from build123d import *

# Parameters (mm, degrees)
BOSS_EXTRU_1_DEPTH      = 12
BOSS_EXTRU_1_DEPTH_BACK = 12
ENL_V_START             = 9
ESQUISSE2_R             = 1
ENL_V_MAT_EXTRU_1_DEPTH = 4
CONG_1_R                = 1
ESQUISSE3_R             = 1
ENL_V_MAT_EXTRU_2_DEPTH = 2.5
ENL_V_START_2           = -2.5
ESQUISSE6_R             = 1
ENL_V_MAT_EXTRU_4_DEPTH = 2.5


with BuildPart() as part:
    # Esquisse1 → Boss.-Extru.1 (new, two sides: drawn at the far end of the back side and taken through both)
    with BuildSketch(Plane.XY.offset(-BOSS_EXTRU_1_DEPTH_BACK)):
        with BuildLine():
            Line((11, -9), (2.692582404, -9))
            ThreePointArc((2.692582404, -9), (0, 5.5), (-2.692582404, -9))
            Line((-2.692582404, -9), (-11, -9))
            Line((-11, -9), (-11, 9))
            Line((-11, 9), (11, 9))
            Line((11, 9), (11, -9))
        make_face()
    extrude(amount=BOSS_EXTRU_1_DEPTH + BOSS_EXTRU_1_DEPTH_BACK)

    # Esquisse2 → Enlèv. mat.-Extru.1 (cut)
    with BuildSketch(Plane(origin=(0, 0, 0), x_dir=(1, 0, 0), z_dir=(0, 1, 0)).offset(ENL_V_START)):
        with Locations(Location((-7, 8, 0), (0, 0, 270))):
            Circle(ESQUISSE2_R)
        with Locations(Location((7, 8, 0), (0, 0, 270))):
            Circle(ESQUISSE2_R)
        with Locations(Location((7, -8, 0), (0, 0, 270))):
            Circle(ESQUISSE2_R)
        with Locations(Location((-7, -8, 0), (0, 0, 270))):
            Circle(ESQUISSE2_R)
    extrude(amount=-ENL_V_MAT_EXTRU_1_DEPTH, mode=Mode.SUBTRACT)

    # Congé1
    cong_1_edges = [part.edges().sort_by_distance(p)[0] for p in [
        (-11, 9, 0),
        (11, 9, 0),
        (11, -9, 0),
        (2.692582404, -9, 0),
        (-2.692582404, -9, 0),
        (-11, -9, 0),
        (0, 5.5, -12),
        (6.846291202, -9, -12),
        (-11, 0, 12),
        (-6.846291202, -9, 12),
        (0, 5.5, 12),
        (6.846291202, -9, 12),
        (11, 0, 12),
        (0, 9, 12),
        (11, 0, -12),
        (0, 9, -12),
        (-11, 0, -12),
        (-6.846291202, -9, -12),
    ]]
    fillet(cong_1_edges, radius=CONG_1_R)

    # Esquisse3 → Enlèv. mat.-Extru.2 (cut)
    with BuildSketch(Plane.ZY.offset(11)):
        with Locations((0, 5.5)):
            Circle(ESQUISSE3_R)
        with Locations((0, -5.5)):
            Circle(ESQUISSE3_R)
    extrude(amount=-ENL_V_MAT_EXTRU_2_DEPTH, mode=Mode.SUBTRACT)

    # Esquisse6 → Enlèv. mat.-Extru.4 (cut)
    with BuildSketch(Plane(origin=(11, 0, 0), x_dir=(0, 0, -1), z_dir=(1, 0, 0)).offset(ENL_V_START_2)):
        with Locations(Location((0, 5.5, 0), (0, 0, 180))):
            Circle(ESQUISSE6_R)
        with Locations(Location((0, -5.5, 0), (0, 0, 180))):
            Circle(ESQUISSE6_R)
    extrude(amount=ENL_V_MAT_EXTRU_4_DEPTH, mode=Mode.SUBTRACT)


solid = part.part
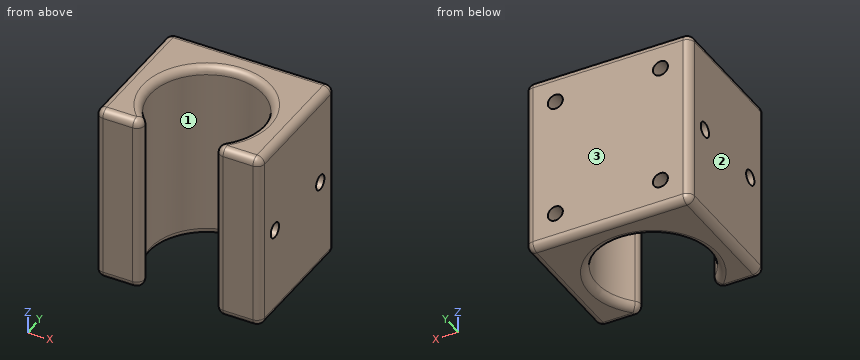
Check sheet for the modelled part. Datum: model origin and axes. Units: mm. Face numbers are marked on the shaded views. Coordinates: 2 decimals unless noted, no trailing zeros. Loops run counter-clockwise (first coordinate to the right, second up) from the corner with the lowest first, then second, coordinate; pieces in that order, holes last. Notation, with made-up numbers: (-27, 36) -> (-6, 36) arc R28 cw to (-6, 67) -> close; hole circle Ø5 at (39, -9.75). An arc over 180 degrees is marked (long way). Write item = value, one per line. Start each with the question number.
1. Section check A-A on x = 0. Record the cut outline in (y, z).
2. Depth check by flat-ended pin: P1, Ø2, axis at x = -5, z = 8, coming from the -Y side; P2, Ø1.6, axis at y = -5.5, z = 0, coming from the -X side; P3, Ø1, axis at x = 7, z = 8, coming from the +Y side; P4, Ø1, axis at x = 0.5, z = -7, coming from the -Y side. Enter the tip coordinate at first touch or a pass-through.
3. Section check B-B on z = 10. Record the cut outline in (x, y), then the cut area to 3 significant figures.
4. Draft check along Y on the marked faces 1, 2 and 3. Enter one of: released by +Y, released by -Y, zero draft, split by the parting line, or undercut.
5. Material ranges on line 1 (Y direction, x = 10.05, z = 0); line 2 (X direction, y = 7.3, z = -8); line 3 (X direction, y = -6.5, z = 4.25), recorded low to high.
Responses:
q1.outline = (5.5, -11) arc R1 ccw to (6.5, -12) -> (8, -12) arc R1 ccw to (9, -11) -> (9, 11) arc R1 ccw to (8, 12) -> (6.5, 12) arc R1 ccw to (5.5, 11) -> close
q2.P1 = -9
q2.P2 = -8.5
q2.P3 = 5
q2.P4 = 5.43
q3.outline = (-11, -8) arc R1 ccw to (-10, -9) -> (-6.02, -9) arc R1 ccw to (-5.31, -7.29) arc R7.5 cw (long way) to (5.31, -7.29) arc R1 ccw to (6.02, -9) -> (10, -9) arc R1 ccw to (11, -8) -> (11, 8) arc R1 ccw to (10, 9) -> (-10, 9) arc R1 ccw to (-11, 8) -> close
q3.area = 217 mm2
q4.face_1 = undercut
q4.face_2 = zero draft
q4.face_3 = released by +Y
q5.line_1 = -9 to -6.5, -4.5 to 4.5, 6.5 to 9
q5.line_2 = -11 to -8, -6 to 6, 8 to 11
q5.line_3 = -11 to -6, 6 to 11
